For this review, take the finished solid that the model builds, in its own axes (mm). A direction names the side the tool comes from. Give positions to 0.01 mm unless a question says otherwise; leave off trailing zeros. Order: outer loops, then holes, each group sorted by start corner. A loop starts at its lowest first (then second) coordinate and runs counter-clockwise, first axis right, second up. Notation, with made-up numbers: (70, -21) - (115, -21) arc R18 cw to (115, -14) - close; hole circle Ø9 at (54.25, 73.5). An arc over 180 degrees is marked (long way). Answer as a JSON object with one key per item and string values. Group by question number.
from build123d import *

# Parameters (mm, degrees)
SKETCH1_W           = 79
SKETCH1_H           = 9
SKETCH1_R           = 2.5
BOSS_EXTRUDE1_DEPTH = 8
SKETCH2_W           = 60
SKETCH2_H           = 6
BOSS_EXTRUDE2_DEPTH = 15
SKETCH3_W           = 1.5
SKETCH3_H           = 1.5
BOSS_EXTRUDE3_DEPTH = 60
SKETCH4_W           = 35
SKETCH4_H           = 6
CUT_EXTRUDE1_DEPTH  = 23
FILLET1_R           = 2.5
FILLET2_R           = 1


with BuildPart() as part:
    # Sketch1 → Boss-Extrude1 (new body)
    with BuildSketch(Plane.XY):
        Rectangle(SKETCH1_W, SKETCH1_H)
        with Locations((-34.5, 0)):
            Circle(SKETCH1_R, mode=Mode.SUBTRACT)
        with Locations((34.5, 0)):
            Circle(SKETCH1_R, mode=Mode.SUBTRACT)
    extrude(amount=BOSS_EXTRUDE1_DEPTH)

    # Sketch2 → Boss-Extrude2 (add)
    with BuildSketch(Plane.XY.offset(8)):
        Rectangle(SKETCH2_W, SKETCH2_H)
    extrude(amount=BOSS_EXTRUDE2_DEPTH)

    # Sketch3 → Boss-Extrude3 (add)
    with BuildSketch(Plane.ZY.offset(30)):
        with Locations((8.75, -3.75)):
            Rectangle(SKETCH3_W, SKETCH3_H)
        with Locations((8.75, 3.75)):
            Rectangle(SKETCH3_W, SKETCH3_H)
    extrude(amount=-BOSS_EXTRUDE3_DEPTH)

    # Sketch4 → Cut-Extrude1 (cut)
    with BuildSketch(Plane(origin=(0, 0, 23), x_dir=(-1, 0, 0), z_dir=(0, 0, -1))):
        Rectangle(SKETCH4_W, SKETCH4_H)
    extrude(amount=CUT_EXTRUDE1_DEPTH, mode=Mode.SUBTRACT)

    # Fillet1
    fillet1_edges = [part.edges().sort_by_distance(p)[0] for p in [
        (39.5, -4.5, 4),
        (-39.5, -4.5, 4),
        (-39.5, 4.5, 4),
        (39.5, 4.5, 4),
        (30, 0, 23),
        (-30, 0, 23),
    ]]
    fillet(fillet1_edges, radius=FILLET1_R)

    # Fillet2
    fillet2_edges = [part.edges().sort_by_distance(p)[0] for p in [
        (0, 4.5, 9.5),
        (-30, 3.75, 9.5),
        (30, 3.75, 9.5),
        (0, -4.5, 9.5),
        (-30, -3.75, 9.5),
        (30, -3.75, 9.5),
        (-22.5, 3, 23),
        (22.5, -3, 23),
        (-17.5, 3, 16.25),
        (17.5, -3, 16.25),
        (-17.5, 0, 23),
        (17.5, 3, 16.25),
        (17.5, 0, 23),
        (-17.5, -3, 16.25),
        (22.5, 3, 23),
        (30, 3, 15),
        (29.267766953, 3, 22.267766953),
        (30, -3, 15),
        (29.267766953, -3, 22.267766953),
        (-22.5, -3, 23),
        (-30, -3, 15),
        (-29.267766953, -3, 22.267766953),
        (-30, 3, 15),
        (-29.267766953, 3, 22.267766953),
    ]]
    fillet(fillet2_edges, radius=FILLET2_R)


solid = part.part
1) For faces 1 (the face through (17.5, 0, 11)), 2 (the face through (30, -1, 14)), 3 (the face through (-37, 1, 8)), list the 3-axis set-ups (+Z, -Z, +X, -X, +Y, -Y) from which the entire face can be reached by the end or side of a thin tool; tool diameter is ignored.
2) Consider section D-D (x = 35). Give the boundary of the cut face in (y, z), plus the area to 3 significant figures.
3) Mouldability with a two-part tool opening along X and no side actions: class faces 4 (the face through (0, 3, 5)), 5 (the face through (37, 1, 8)), 6 (the face through (29.287, 0.028, 22.248)), 7 (the face through (-39.5, 0, 4)) as released by +X, released by -X, zero draft, split by the parting line, or undercut.
4) Consider section A-A (x = -15). Give the boundary of the cut face in (y, z), plus the area to 3 significant figures.
5) Consider section B-B (z = 13.5). Give the boundary of the cut face in (x, y), plus the area to 3 significant figures.
6) For pin 1 (1.5 mm diameter, centred on y = -3.5, z = 4.5, fed in from +X); pin 2 (11.5 mm diameter, centred on x = 24.5, z = 18, fed in from -Y); pin 3 (5 mm diameter, centred on x = 26, z = 15, fed in from +Y); pin 4 (3 mm diameter, centred on x = 34.5, y = 0, fed in from +Z), all flat-tipped, find the tip position at first contact; note any pin that passes through.
7) Consider section C-C (x = -34.5). Give the boundary of the cut face in (y, z), plus the area to 3 significant figures.
8) For line 1 (Y direction, x = -34.5, z = 2.75); line 2 (X direction, y = 1, z = 10.5); line 3 (Y direction, x = -10, z = 6.5), list the stretches that pass through material, from the lowest coordinate up.
Result set:
{
 "1": {"face 1": "+Z, -Z", "face 2": "+Z, +X, +Y, -Y", "face 3": "+Z, -X, +Y, -Y"},
 "2": {"outline": "(-4.5, 0) - (-2.45, 0) - (-2.45, 8) - (-4.5, 8) - close; (2.45, 0) - (4.5, 0) - (4.5, 8) - (2.45, 8) - close", "area": "32.8 mm2"},
 "3": {"face 4": "undercut", "face 5": "zero draft", "face 6": "released by +X", "face 7": "released by -X"},
 "4": {"outline": "(-4.5, 0) - (-3, 0) - (-3, 9.5) - (-3.5, 9.5) arc R1 ccw to (-4.5, 8.5) - close; (3, 0) - (4.5, 0) - (4.5, 8.5) arc R1 ccw to (3.5, 9.5) - (3, 9.5) - close", "area": "28.1 mm2"},
 "5": {"outline": "(-30, -2) arc R1 ccw to (-29, -3) - (-18.5, -3) arc R1 ccw to (-17.5, -2) - (-17.5, 2) arc R1 ccw to (-18.5, 3) - (-29, 3) arc R1 ccw to (-30, 2) - close; (17.5, -2) arc R1 ccw to (18.5, -3) - (29, -3) arc R1 ccw to (30, -2) - (30, 2) arc R1 ccw to (29, 3) - (18.5, 3) arc R1 ccw to (17.5, 2) - close", "area": "148 mm2"},
 "6": {"pin 1": "stops at x = 39.38", "pin 2": "stops at y = -3", "pin 3": "stops at y = 3", "pin 4": "passes through"},
 "7": {"outline": "(-4.5, 0) - (-2.5, 0) - (-2.5, 8) - (-4.5, 8) - close; (2.5, 0) - (4.5, 0) - (4.5, 8) - (2.5, 8) - close", "area": "32.0 mm2"},
 "8": {"line 1": "y = -4.5 to -2.5, 2.5 to 4.5", "line 2": "x = -30 to -17.5, 17.5 to 30", "line 3": "y = -4.5 to -3, 3 to 4.5"}
}
